```python
from build123d import *

# Parameters (mm, degrees)
SKETCH2_W               = 190.5
SKETCH2_H               = 177.8
BOSS_EXTRUDE1_DEPTH     = 5.08
CHAMFER1_SIZE           = 25.4
BOSS_EXTRUDE3_DEPTH     = 68.42
SKETCH5_R               = 9
SKETCH5_R_2             = 1.5
CUT_EXTRUDE1_DEPTH      = 231.530019737
SKETCH10_W              = 177.8
SKETCH10_H              = 73.5
BOSS_EXTRUDE6_DEPTH     = 30
CHAMFER3_SIZE           = 25.4
CUT_EXTRUDE2_DEPTH      = 68.42
BOSS_EXTRUDE7_START     = 38.1
BOSS_EXTRUDE7_DEPTH     = 12.7
SKETCH13_W              = 15.24
SKETCH13_H              = 12.7
BOSS_EXTRUDE8_DEPTH     = 7
SKETCH14_R              = 2.5
CUT_EXTRUDE3_DEPTH      = 10
MIRROR4_COPY_1_SKETCH_W = 15.24
MIRROR4_COPY_1_SKETCH_H = 12.7
MIRROR4_COPY_1_DEPTH    = 7
MIRROR4_COPY_2_SKETCH_R = 2.5
MIRROR4_COPY_2_DEPTH    = 10
SKETCH17_W              = 6
SKETCH17_H              = 6
SKETCH17_R              = 1.35
BOSS_EXTRUDE9_DEPTH     = 3
SKETCH18_W              = 5.5
SKETCH18_H              = 5.5
SKETCH18_R              = 1.5
BOSS_EXTRUDE10_DEPTH    = 3
SKETCH19_W              = 6
SKETCH19_H              = 6
SKETCH19_R              = 1.5
BOSS_EXTRUDE11_DEPTH    = 3
SKETCH19_2_R            = 1.5
CUT_EXTRUDE5_DEPTH      = 10
SKETCH17_2_R            = 1.35
CUT_EXTRUDE6_DEPTH      = 10
SKETCH18_2_R            = 1.5
CUT_EXTRUDE7_DEPTH      = 10
SKETCH20_R              = 7.5
CUT_EXTRUDE8_DEPTH      = 10
SKETCH20_3_R            = 10.5
SKETCH20_3_R_2          = 7.5
CUT_EXTRUDE9_DEPTH      = 4
CHAMFER4_SIZE           = 0.5
SKETCH18_3_R            = 1.5
CUT_EXTRUDE10_DEPTH     = 10
SKETCH22_R              = 1.5
CUT_EXTRUDE11_DEPTH     = 10


with BuildPart() as part:
    # Sketch2 → Boss-Extrude1 (new body)
    with BuildSketch(Plane(origin=(0, 0, 0), x_dir=(1, 0, 0), z_dir=(0, 1, 0))):
        with Locations((-31.75, -12.7)):
            Rectangle(SKETCH2_W, SKETCH2_H)
    extrude(amount=BOSS_EXTRUDE1_DEPTH)

    # Chamfer1
    chamfer1_edges = [part.edges().sort_by_distance(p)[0] for p in [
        (-127, 2.54, -76.2),
        (-127, 2.54, 101.6),
    ]]
    chamfer(chamfer1_edges, length=CHAMFER1_SIZE)

    # Sketch4 → Boss-Extrude3 (add)
    with BuildSketch(Plane(origin=(0, 5.08, 0), x_dir=(1, 0, 0), z_dir=(0, 1, 0))):
        Polygon((57.15, 69.85), (-98.969743879, 69.85), (-120.65, 48.169743879), (-120.65, -73.569743879), (-98.969743879, -95.25), (57.15, -95.25), (63.5, -95.25), (63.5, -101.6), (-101.6, -101.6), (-127, -76.2), (-127, 50.8), (-101.6, 76.2), (63.5, 76.2), (63.5, 69.85), align=None)
    extrude(amount=BOSS_EXTRUDE3_DEPTH)

    # Sketch5 → Cut-Extrude1 (cut, through all)
    with BuildSketch(Plane.XY.offset(101.6)):
        with Locations((-50.8, 31.75)):
            Circle(SKETCH5_R)
        with Locations((-50.8, 47.25)):
            Circle(SKETCH5_R_2)
        with Locations((-37.376606241, 39.5)):
            Circle(SKETCH5_R_2)
        with Locations((-37.376606241, 24)):
            Circle(SKETCH5_R_2)
        with Locations((-50.8, 16.25)):
            Circle(SKETCH5_R_2)
        with Locations((-64.223393759, 24)):
            Circle(SKETCH5_R_2)
        with Locations((-64.223393759, 39.5)):
            Circle(SKETCH5_R_2)
    extrude(amount=-CUT_EXTRUDE1_DEPTH, mode=Mode.SUBTRACT)

    # Sketch10 → Boss-Extrude6 (add)
    with BuildSketch(Plane(origin=(63.5, 0, 0), x_dir=(0, 0, -1), z_dir=(1, 0, 0))):
        with Locations((-12.7, 36.75)):
            Rectangle(SKETCH10_W, SKETCH10_H)
    extrude(amount=BOSS_EXTRUDE6_DEPTH)

    # Chamfer3
    chamfer3_edges = [part.edges().sort_by_distance(p)[0] for p in [
        (93.5, 36.75, 101.6),
        (93.5, 36.75, -76.2),
    ]]
    chamfer(chamfer3_edges, length=CHAMFER3_SIZE)

    # Sketch11 → Cut-Extrude2 (cut)
    with BuildSketch(Plane(origin=(0, 73.5, 0), x_dir=(1, 0, 0), z_dir=(0, 1, 0))):
        Polygon((85.757180746, -72.992819254), (85.757180746, 47.592819254), (63.5, 69.85), (63.5, -95.25), align=None)
    extrude(amount=-CUT_EXTRUDE2_DEPTH, mode=Mode.SUBTRACT)

    # Sketch12 → Boss-Extrude7 (add)
    with BuildSketch(Plane(origin=(0, 0, 95.25), x_dir=(-1, 0, 0), z_dir=(0, 0, -1)).offset(BOSS_EXTRUDE7_START)):
        with BuildLine():
            Line((25.8, 5.08), (75.8, 5.08))
            Line((75.8, 5.08), (75.8, 31.75))
            Line((75.8, 31.75), (69.8, 31.75))
            ThreePointArc((69.8, 31.75), (50.8, 12.75), (31.8, 31.75))
            Line((31.8, 31.75), (25.8, 31.75))
            Line((25.8, 31.75), (25.8, 5.08))
        make_face()
    boss_extrude7 = extrude(amount=BOSS_EXTRUDE7_DEPTH)

    # Sketch13 → Boss-Extrude8 (add)
    with BuildSketch(Plane(origin=(0, 31.75, 0), x_dir=(1, 0, 0), z_dir=(0, 1, 0))):
        with Locations((-24.18, -50.8)):
            Rectangle(SKETCH13_W, SKETCH13_H)
    boss_extrude8 = extrude(amount=-BOSS_EXTRUDE8_DEPTH)

    # Sketch14 → Cut-Extrude3 (cut)
    with BuildSketch(Plane(origin=(0, 31.75, 0), x_dir=(1, 0, 0), z_dir=(0, 1, 0))):
        with Locations(Location((-20.37, -50.8, 0), (0, 0, 270))):
            Circle(SKETCH14_R)
    cut_extrude3 = extrude(amount=-CUT_EXTRUDE3_DEPTH, mode=Mode.SUBTRACT)

    # Mirror2: Boss-Extrude8 across plane
    add(boss_extrude8.mirror(Plane.ZY.offset(50.8)))

    # Mirror3: Cut-Extrude3 across plane
    add(cut_extrude3.mirror(Plane.ZY.offset(50.8)), mode=Mode.SUBTRACT)

    # Mirror4: Boss-Extrude7, Boss-Extrude8, Cut-Extrude3 across plane
    add(boss_extrude7.mirror(Plane.XY.offset(12.7)))
    add(boss_extrude8.mirror(Plane.XY.offset(12.7)))
    add(cut_extrude3.mirror(Plane.XY.offset(12.7)), mode=Mode.SUBTRACT)

    # Mirror4 copy 1 sketch → Mirror4 copy 1 (add)
    with BuildSketch(Plane(origin=(-101.6, 31.75, 25.4), x_dir=(-1, 0, 0), z_dir=(0, 1, 0))):
        with Locations((-24.18, -50.8)):
            Rectangle(MIRROR4_COPY_1_SKETCH_W, MIRROR4_COPY_1_SKETCH_H)
    extrude(amount=-MIRROR4_COPY_1_DEPTH)

    # Mirror4 copy 2 sketch → Mirror4 copy 2 (cut)
    with BuildSketch(Plane(origin=(-101.6, 31.75, 25.4), x_dir=(-1, 0, 0), z_dir=(0, 1, 0))):
        with Locations(Location((-20.37, -50.8, 0), (0, 0, 270))):
            Circle(MIRROR4_COPY_2_SKETCH_R)
    extrude(amount=-MIRROR4_COPY_2_DEPTH, mode=Mode.SUBTRACT)

    # Sketch17 → Boss-Extrude9 (add)
    with BuildSketch(Plane(origin=(0, 5.08, 0), x_dir=(1, 0, 0), z_dir=(0, 1, 0))):
        with Locations((7.5, 64.85)):
            Rectangle(SKETCH17_W, SKETCH17_H)
        with Locations(Location((7.5, 64.85, 0), (0, 0, 270))):
            Circle(SKETCH17_R, mode=Mode.SUBTRACT)
        with Locations((56.5, 64.85)):
            Rectangle(SKETCH17_W, SKETCH17_H)
        with Locations(Location((56.5, 64.85, 0), (0, 0, 270))):
            Circle(SKETCH17_R, mode=Mode.SUBTRACT)
        with Locations((7.5, 6.85)):
            Rectangle(SKETCH17_W, SKETCH17_H)
        with Locations(Location((7.5, 6.85, 0), (0, 0, 270))):
            Circle(SKETCH17_R, mode=Mode.SUBTRACT)
        with Locations((56.5, 6.85)):
            Rectangle(SKETCH17_W, SKETCH17_H)
        with Locations(Location((56.5, 6.85, 0), (0, 0, 270))):
            Circle(SKETCH17_R, mode=Mode.SUBTRACT)
    extrude(amount=BOSS_EXTRUDE9_DEPTH)

    # Sketch18 → Boss-Extrude10 (add)
    with BuildSketch(Plane(origin=(0, 5.08, 0), x_dir=(1, 0, 0), z_dir=(0, 1, 0))):
        with Locations((-105.65, 48.95)):
            Rectangle(SKETCH18_W, SKETCH18_H)
        with Locations(Location((-105.65, 48.95, 0), (0, 0, 270))):
            Circle(SKETCH18_R, mode=Mode.SUBTRACT)
        with Locations((-89.65, 18.95)):
            Rectangle(SKETCH18_W, SKETCH18_H)
        with Locations(Location((-89.65, 18.95, 0), (0, 0, 270))):
            Circle(SKETCH18_R, mode=Mode.SUBTRACT)
        with Locations((-105.65, 18.95)):
            Rectangle(SKETCH18_W, SKETCH18_H)
        with Locations(Location((-105.65, 18.95, 0), (0, 0, 270))):
            Circle(SKETCH18_R, mode=Mode.SUBTRACT)
        with Locations((-89.65, 48.95)):
            Rectangle(SKETCH18_W, SKETCH18_H)
        with Locations(Location((-89.65, 48.95, 0), (0, 0, 270))):
            Circle(SKETCH18_R, mode=Mode.SUBTRACT)
    extrude(amount=BOSS_EXTRUDE10_DEPTH)

    # Sketch19 → Boss-Extrude11 (add)
    with BuildSketch(Plane(origin=(0, 5.08, 0), x_dir=(1, 0, 0), z_dir=(0, 1, 0))):
        with Locations((11.057180746, -49.55)):
            Rectangle(SKETCH19_W, SKETCH19_H)
        with Locations(Location((11.057180746, -49.55, 0), (0, 0, 270))):
            Circle(SKETCH19_R, mode=Mode.SUBTRACT)
        with Locations((47.757180746, -49.55)):
            Rectangle(SKETCH19_W, SKETCH19_H)
        with Locations(Location((47.757180746, -49.55, 0), (0, 0, 270))):
            Circle(SKETCH19_R, mode=Mode.SUBTRACT)
        with Locations((11.057180746, -86.25)):
            Rectangle(SKETCH19_W, SKETCH19_H)
        with Locations(Location((11.057180746, -86.25, 0), (0, 0, 270))):
            Circle(SKETCH19_R, mode=Mode.SUBTRACT)
        with Locations((47.757180746, -86.25)):
            Rectangle(SKETCH19_W, SKETCH19_H)
        with Locations(Location((47.757180746, -86.25, 0), (0, 0, 270))):
            Circle(SKETCH19_R, mode=Mode.SUBTRACT)
    extrude(amount=BOSS_EXTRUDE11_DEPTH)

    # Sketch19_2 → Cut-Extrude5 (cut)
    with BuildSketch(Plane(origin=(0, 5.08, 0), x_dir=(1, 0, 0), z_dir=(0, 1, 0))):
        with Locations(Location((11.057180746, -49.55, 0), (0, 0, 270))):
            Circle(SKETCH19_2_R)
        with Locations(Location((47.757180746, -49.55, 0), (0, 0, 270))):
            Circle(SKETCH19_2_R)
        with Locations(Location((47.757180746, -86.25, 0), (0, 0, 270))):
            Circle(SKETCH19_2_R)
        with Locations(Location((11.057180746, -86.25, 0), (0, 0, 270))):
            Circle(SKETCH19_2_R)
    extrude(amount=-CUT_EXTRUDE5_DEPTH, mode=Mode.SUBTRACT)

    # Sketch17_2 → Cut-Extrude6 (cut)
    with BuildSketch(Plane(origin=(0, 5.08, 0), x_dir=(1, 0, 0), z_dir=(0, 1, 0))):
        with Locations(Location((7.5, 64.85, 0), (0, 0, 270))):
            Circle(SKETCH17_2_R)
        with Locations(Location((56.5, 64.85, 0), (0, 0, 270))):
            Circle(SKETCH17_2_R)
        with Locations(Location((56.5, 6.85, 0), (0, 0, 270))):
            Circle(SKETCH17_2_R)
        with Locations(Location((7.5, 6.85, 0), (0, 0, 270))):
            Circle(SKETCH17_2_R)
    extrude(amount=-CUT_EXTRUDE6_DEPTH, mode=Mode.SUBTRACT)

    # Sketch18_2 → Cut-Extrude7 (cut)
    with BuildSketch(Plane(origin=(0, 5.08, 0), x_dir=(1, 0, 0), z_dir=(0, 1, 0))):
        with Locations(Location((-89.65, 18.95, 0), (0, 0, 270))):
            Circle(SKETCH18_2_R)
        with Locations(Location((-105.65, 48.95, 0), (0, 0, 270))):
            Circle(SKETCH18_2_R)
    extrude(amount=-CUT_EXTRUDE7_DEPTH, mode=Mode.SUBTRACT)

    # Sketch20 → Cut-Extrude8 (cut)
    with BuildSketch(Plane(origin=(93.5, 0, 0), x_dir=(0, 0, -1), z_dir=(1, 0, 0))):
        with Locations((-12.7, 20)):
            Circle(SKETCH20_R)
    extrude(amount=-CUT_EXTRUDE8_DEPTH, mode=Mode.SUBTRACT)

    # Sketch20_3 → Cut-Extrude9 (cut)
    with BuildSketch(Plane(origin=(93.5, 0, 0), x_dir=(0, 0, -1), z_dir=(1, 0, 0))):
        with Locations((-12.7, 20)):
            Circle(SKETCH20_3_R)
        with Locations((-12.7, 20)):
            Circle(SKETCH20_3_R_2, mode=Mode.SUBTRACT)
    extrude(amount=-CUT_EXTRUDE9_DEPTH, mode=Mode.SUBTRACT)

    # Chamfer4
    chamfer4_edges = [part.edges().sort_by_distance(p)[0] for p in [
        (93.5, 20, 23.2),
    ]]
    chamfer(chamfer4_edges, length=CHAMFER4_SIZE)

    # Sketch18_3 → Cut-Extrude10 (cut)
    with BuildSketch(Plane(origin=(0, 5.08, 0), x_dir=(1, 0, 0), z_dir=(0, 1, 0))):
        with Locations(Location((-89.65, 48.95, 0), (0, 0, 270))):
            Circle(SKETCH18_3_R)
        with Locations(Location((-105.65, 18.95, 0), (0, 0, 270))):
            Circle(SKETCH18_3_R)
    extrude(amount=-CUT_EXTRUDE10_DEPTH, mode=Mode.SUBTRACT)

    # Sketch22 → Cut-Extrude11 (cut)
    with BuildSketch(Plane(origin=(93.5, 0, 0), x_dir=(0, 0, -1), z_dir=(1, 0, 0))):
        with Locations((-42.7, 43.5)):
            Circle(SKETCH22_R)
        with Locations((17.3, 43.5)):
            Circle(SKETCH22_R)
        with Locations((-42.7, 13.5)):
            Circle(SKETCH22_R)
        with Locations((17.3, 13.5)):
            Circle(SKETCH22_R)
    extrude(amount=-CUT_EXTRUDE11_DEPTH, mode=Mode.SUBTRACT)


solid = part.part
```
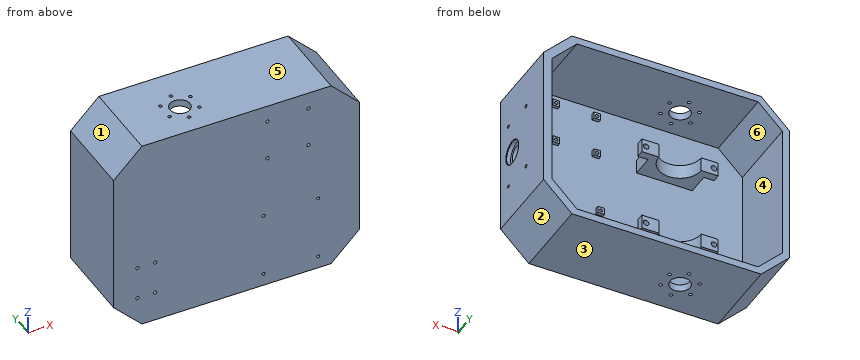
CAD build for the part. Positions are in the model's coordinates, mm. Face numbers are marked on the shaded views. A direction names the side the tool comes from. Round coordinates to 2 decimals unless told otherwise and drop trailing zeros. Loops run counter-clockwise (first coordinate to the right, second up) from the corner with the lowest first, then second, coordinate; pieces in that order, holes last. Notation, with made-up numbers: M 9.25,70 L 15.25,70 A22 cw 15.25,98 Z; hole C 57.5,2.5 d10. An arc over 180 degrees is marked long. Return JSON: item names as keys, results as strings. Group by question number.
(1) Tool access for the marked faces 5 and 6: list every direction of +Z, -Z, +X, -X, +Y, -Y with a clear straight run to the whole face (end or side of a thin tool).
(2) Wall check: probe 1 along Z at (x, y) = (-89.65, 3.15); probe 2 along Z at (x, y) = (-74, 24.5); probe 3 along Y at (x, z) = (-78, 46.5). Give the ranges that are in metal, low to high. Write a range as [from, to].
(3) Saw through at C-C, the plane z = -25.4. List the corners of the cut face in (x, y).
(4) Drop flat-ended pins along their axis: P1, Ø8, axis at x = -96.5, z = 3, coming from the -Y side; P2, Ø1, axis at x = -12.5, z = 56, coming from the +Y side; P3, Ø1.5, axis at y = 6, z = -66, coming from the -X side; P4, Ø4.5, axis at x = 56.5, z = -64.85, coming from the +Y side. Give the stop position or say it passes through.
(5) Saw through at A-A, the plane y = 59.5. List the corners of the cut face in (x, z), and give its area (3 significant figures).
(6) Mould opens along X. For the marked faces 1, 2, 3 and 4 say: +X half, -X half, draft (parallel to the pull), parting line (faces both ways), or undercut.
(7) Saw through at B-B, the plane x = -81.23. List the corners of the cut face in (y, z).
(8) Saw through at D-D, the plane z = 70. List the corners of the cut face in (x, y).
Answer list:
{
 "1": {"face 5": "+Z, +X, -X, +Y, -Y", "face 6": "+Y"},
 "2": {"probe 1": "[-76.2, -50.45], [-47.45, -20.45], [-17.45, 101.6]", "probe 2": "[-76.2, -69.85], [-31.75, -19.05], [44.45, 57.15], [95.25, 101.6]", "probe 3": "[0, 5.08], [24.75, 31.75]"},
 "3": {"outline": "M -127,0 L 93.5,0 L 93.5,73.5 L 85.76,73.5 L 85.76,5.08 L -25.8,5.08 L -25.8,24.75 L -22.87,24.75 L -22.87,31.75 L -31.8,31.75 A19 cw -69.8,31.75 L -78.73,31.75 L -78.73,24.75 L -75.8,24.75 L -75.8,5.08 L -120.65,5.08 L -120.65,73.5 L -127,73.5 Z; M -85.04,24.75 L -83.73,24.75 L -83.73,31.75 L -85.04,31.75 Z; M -17.87,24.75 L -16.56,24.75 L -16.56,31.75 L -17.87,31.75 Z"},
 "4": {"P1": "y = 0", "P2": "y = 5.08", "P3": "x = -112.55", "P4": "y = 8.08"},
 "5": {"outline": "M -127,-50.8 L -101.6,-76.2 L 68.1,-76.2 L 93.5,-50.8 L 93.5,76.2 L 68.1,101.6 L -101.6,101.6 L -127,76.2 Z; hole M -120.65,-48.17 L -98.97,-69.85 L 63.5,-69.85 L 85.76,-47.59 L 85.76,72.99 L 63.5,95.25 L -98.97,95.25 L -120.65,73.57 Z", "area": "4,800 mm2"},
 "6": {"face 1": "-X half", "face 2": "+X half", "face 3": "draft", "face 4": "undercut"},
 "7": {"outline": "M 0,-76.2 L 73.5,-76.2 L 73.5,-69.85 L 5.08,-69.85 L 5.08,95.25 L 73.5,95.25 L 73.5,101.6 L 0,101.6 Z; M 24.75,-31.75 L 31.75,-31.75 L 31.75,-27.9 L 24.75,-27.9 Z; M 24.75,-22.9 L 31.75,-22.9 L 31.75,-19.05 L 24.75,-19.05 Z; M 24.75,44.45 L 31.75,44.45 L 31.75,48.3 L 24.75,48.3 Z; M 24.75,53.3 L 31.75,53.3 L 31.75,57.15 L 24.75,57.15 Z"},
 "8": {"outline": "M -127,0 L 93.5,0 L 93.5,73.5 L 85.76,73.5 L 85.76,5.08 L -120.65,5.08 L -120.65,73.5 L -127,73.5 Z"}
}
